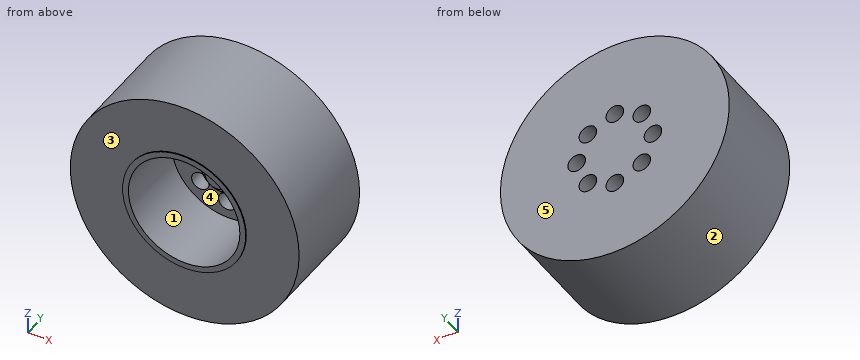
from build123d import *

# Parameters (mm, degrees)
F0_R      = 19.5
F1_DEPTH  = 17
F2_R      = 9.5
F3_DEPTH  = 12
F4_R      = 10.5
F4_R_2    = 9.5
F5_DEPTH  = 0.15
F6_R      = 2
F7_DEPTH  = 3
F8_R      = 3.5
F8_R_2    = 2
F9_DEPTH  = 1.7
F10_R     = 0.5
F11_DEPTH = 0.25
F12_R     = 1.5
F13_DEPTH = 25


with BuildPart() as f1:
    # F0 (on Front) → F1 (new body)
    with BuildSketch(Plane.XZ):
        Circle(F0_R)
    extrude(amount=F1_DEPTH)

    # F2 (on face) → F3 (cut)
    with BuildSketch(Plane.XZ.offset(17)):
        Circle(F2_R)
    extrude(amount=-F3_DEPTH, mode=Mode.SUBTRACT)

    # F4 (on face) → F5 (join)
    with BuildSketch(Plane.XZ.offset(17)):
        Circle(F4_R)
        Circle(F4_R_2, mode=Mode.SUBTRACT)
    extrude(amount=F5_DEPTH)

    # F6 (on face) → F7 (join)
    with BuildSketch(Plane.XZ.offset(5)):
        Circle(F6_R)
    extrude(amount=F7_DEPTH)

    # F8 (on face) → F9 (join)
    with BuildSketch(Plane.XZ.offset(5)):
        Circle(F8_R)
        Circle(F8_R_2, mode=Mode.SUBTRACT)
    extrude(amount=F9_DEPTH)

    # F10 (on face) → F11 (join)
    with BuildSketch(Plane.XZ.offset(6.7)):
        with Locations((0, 2.75)):
            Circle(F10_R)
        with Locations((1.6164094438, 2.2247967345)):
            Circle(F10_R)
        with Locations((2.6154054198, -0.8497967345)):
            Circle(F10_R)
        with Locations((1.6164094438, -2.2247967345)):
            Circle(F10_R)
        with Locations((0, -2.75)):
            Circle(F10_R)
        with Locations((2.6154054198, 0.8497967345)):
            Circle(F10_R)
        with Locations((-1.6164094438, -2.2247967345)):
            Circle(F10_R)
        with Locations((-2.6154054198, -0.8497967345)):
            Circle(F10_R)
        with Locations((-2.6154054198, 0.8497967345)):
            Circle(F10_R)
        with Locations((-1.6164094438, 2.2247967345)):
            Circle(F10_R)
    extrude(amount=F11_DEPTH)

    # F12 (on face) → F13 (cut)
    with BuildSketch(Plane.XZ.offset(5)):
        with Locations((0, 6.5)):
            Circle(F12_R)
        with Locations((4.5961940777, 4.5961940777)):
            Circle(F12_R)
        with Locations((6.5, 0)):
            Circle(F12_R)
        with Locations((-4.5961940777, 4.5961940777)):
            Circle(F12_R)
        with Locations((-6.5, 0)):
            Circle(F12_R)
        with Locations((-4.5961940777, -4.5961940777)):
            Circle(F12_R)
        with Locations((4.5961940777, -4.5961940777)):
            Circle(F12_R)
        with Locations((0, -6.5)):
            Circle(F12_R)
    extrude(amount=-F13_DEPTH, mode=Mode.SUBTRACT)


solid = f1.part
Here's how the part is built. I have some questions about the finished solid (model axes, mm). Face numbers are marked on the shaded views. A direction names the side the tool comes from. Give positions to 0.01 mm unless a question says otherwise; leave off trailing zeros. Order: outer loops, then holes, each group sorted by start corner. A loop starts at its lowest first (then second) coordinate and runs counter-clockwise, first axis right, second up. Notation, with made-up numbers: (-21.75, 3) -> (3.25, 3) arc R32 cw to (3.25, 29) -> close; hole circle Ø9 at (-30, 68.5). An arc over 180 degrees is marked (long way). One line per item, written item: value. Start each with the question number.
1. Imagine slicing it at A-A, the plane x = 0. Count the separate pieces of the cut face and the enclosed holes in it, plus the area to 3 significant figures.
2. We'd pull the mould along X, two halves only. Please class the marked faces 1, 2 and 3: released by +X, released by -X, zero draft, split by the parting line, or undercut.
3. I need wall thicknesses on probe 1 along Z at (x, y) = (0, -1); probe 2 along Y at (x, z) = (9, -17); probe 3 along Y at (x, z) = (-0.5, -1). Which ranges of each line are inside material? Lowest first, please. Write a range as from..to.
4. Imagine slicing it at D-D, the plane x = -4. List the corners of the cut face in (y, z) for me, plus the area to 3 significant figures.
5. Imagine slicing it at B-B, the plane z = -5.5. List the corners of the cut face in (x, y) for me.
6. For the marked faces 4 and 5, which set-ups out of +Z, -Z, +X, -X, +Y, -Y let a thin tool reach every point of the face, with its end or its side?
7. Will these pins go through, and if not, where does the flat tip stop? pin 1 Ø5.5 at (x, z) = (2, 2) entering from -Y; pin 2 Ø1 at (y, z) = (-3.5, -11.5) entering from -X; pin 3 Ø0.8 at (x, z) = (-1.5, 2.5) entering from -Y; pin 4 Ø1.8 at (x, z) = (-6.5, 0) entering from +Y.
8. Imagine slicing it at C-C, the plane y = -16. List the corners of the cut face in (x, z) for me, plus the area to 3 significant figures.
Values follow:
1. separate pieces: 3
1. enclosed holes: 0
1. area: 423 mm2
2. face 1: undercut
2. face 2: split by the parting line
2. face 3: zero draft
3. probe 1: z = -19.5..-8, -5..5, 8..19.5
3. probe 2: y = -17..0
3. probe 3: y = -8..0
4. outline: (-17.15, -9.71) -> (-17, -9.71) -> (-17, -19.09) -> (0, -19.09) -> (0, -5.97) -> (-5, -5.97) -> (-5, -8.62) -> (-17.15, -8.62) -> close; (-17.15, 8.62) -> (-5, 8.62) -> (-5, 5.97) -> (0, 5.97) -> (0, 19.09) -> (-17, 19.09) -> (-17, 9.71) -> (-17.15, 9.71) -> close; (-5, -3.22) -> (0, -3.22) -> (0, 3.22) -> (-5, 3.22) -> close
4. area: 415 mm2
5. outline: (-18.71, -17) -> (-8.94, -17) -> (-8.94, -17.15) -> (-7.75, -17.15) -> (-7.75, -5) -> (-5.79, -5) -> (-5.79, 0) -> (-18.71, 0) -> close; (-3.4, -5) -> (-1.12, -5) -> (-1.12, 0) -> (-3.4, 0) -> close; (1.12, -5) -> (3.4, -5) -> (3.4, 0) -> (1.12, 0) -> close; (5.79, -5) -> (7.75, -5) -> (7.75, -17.15) -> (8.94, -17.15) -> (8.94, -17) -> (18.71, -17) -> (18.71, 0) -> (5.79, 0) -> close
6. face 4: -Y
6. face 5: +Z, -Z, +X, -X, +Y
7. pin 1: stops at y = -8
7. pin 2: stops at x = -16.1
7. pin 3: stops at y = -6.95
7. pin 4: passes through
8. outline: circle Ø39 at (0, 0); hole circle Ø19 at (0, 0)
8. area: 911 mm2
